Read the model definition and answer for the solid it produces. Units are mm, in the model's axes. Coordinates: 2 decimals unless noted, no trailing zeros. Loops run counter-clockwise (first coordinate to the right, second up) from the corner with the lowest first, then second, coordinate; pieces in that order, holes last.
Q1. Section B-B (z = 4.5) is taken. Give the vertices of the cut face in (x, y) (3 decimals).
Q2. Section A-A (y = 2) is taken. Give the vertices of the cut face in (x, z).
Q3. Straight lines are drawn through the part: line 1 (X direction, y = -2, z = 3.75); line 2 (Z direction, x = 11, y = -1) (3 decimals); line 3 (X direction, y = 1, z = 3.5). For each, find the intervals that lie inside material, in ascending order.
Q4. Flat-ended cylindrical pins translate along their axes: P1, Ø3, axis at x = 8.5, y = 2.5, coming from the -Z side; P2, Ø2, axis at y = -1, z = 10.5, coming from the +X side. Find the tip coordinate at first contact, or state that the pin passes through.
Q5. Section D-D (x = 11.75) is taken. Give the vertices of the cut face in (y, z) (3 decimals), then the cut area to 3 significant figures.
Q6. Section C-C (z = 3.5) is taken. Give the vertices of the cut face in (x, y) (3 decimals).
Q7. The mould has two halves that part along X. Classify faces 1 (the face through (0, -0.044, 11.203)), 2 (the face through (23.637, 0, 7)), 3 (the face through (21.75, 0.04, 2.99)), 4 (the face through (11, 3.175, 7)): pulls with the +X half, pulls with the -X half, needs draft (parallel to the pull), parting line crosses it, or undercut.
from build123d import *

# Parameters (mm, degrees)
F1_DEPTH = 3.175
F2_R     = 3.81


with BuildPart() as f1:
    # F0 (on Front) → F1 (new body, symmetric)
    with BuildSketch(Plane.XZ):
        with BuildLine():
            ThreePointArc((23.63662, 14.987046), (10.93662, 9.954885), (-1.76338, 14.987046))
            Line((-1.76338, 14.987046), (-1.76338, -4.062954))
            ThreePointArc((-1.76338, -4.062954), (10.93662, 4.934133), (23.63662, -4.062954))
            Line((23.63662, -4.062954), (23.63662, 14.987046))
        make_face()
    extrude(amount=F1_DEPTH, both=True)

    # F2
    f2_edges = [f1.edges().sort_by_distance(p)[0] for p in [
        (23.63662, 0, 14.987046),
        (23.63662, 0, -4.062954),
        (-1.76338, 0, -4.062954),
        (-1.76338, 0, 14.987046),
    ]]
    fillet(f2_edges, radius=F2_R)


solid = f1.part
Numbers:
1. outline: (-1.322, -3.175) - (7.545, -3.175) - (7.545, 3.175) - (-1.322, 3.175) - close; (14.328, -3.175) - (23.195, -3.175) - (23.195, 3.175) - (14.328, 3.175) - close
2. outline: (-1.76, 6.28) arc R3.81 ccw to (4.01, 3.01) arc R13.46 cw to (17.87, 3.01) arc R3.81 ccw to (23.64, 6.28) - (23.64, 7.99) arc R3.81 ccw to (18.31, 11.48) arc R18.54 cw to (3.56, 11.48) arc R3.81 ccw to (-1.76, 7.99) - close
3. line 1: x = -0.8 to 5.42, 16.46 to 22.67
3. line 2: z = 4.934 to 9.955
3. line 3: x = -0.56 to 4.89, 16.98 to 22.43
4. P1: stops at z = 4.35
4. P2: stops at x = 23.32
5. outline: (-3.175, 4.91) - (3.175, 4.91) - (3.175, 9.973) - (-3.175, 9.973) - close
5. area: 32.2 mm2
6. outline: (-0.558, -3.175) - (4.89, -3.175) - (4.89, 3.175) - (-0.558, 3.175) - close; (16.983, -3.175) - (22.431, -3.175) - (22.431, 3.175) - (16.983, 3.175) - close
7. face 1: undercut
7. face 2: pulls with the +X half
7. face 3: undercut
7. face 4: needs draft
